Geometry: final body of the model. Coordinates: model frame, mm. A direction names the side the tool comes from. Coordinates: 2 decimals unless noted, no trailing zeros. Order: outer loops, then holes, each group sorted by start corner. A loop starts at its lowest first (then second) coordinate and runs counter-clockwise, first axis right, second up. Notation, with made-up numbers: (38, 22) - (69, 22) arc R30 ccw to (69, 48) - close; hole circle Ø11 at (-2, 83.5). An arc over 180 degrees is marked (long way). Use a Markdown table: item, result. Add a question column.
```python
from build123d import *

# Parameters (mm, degrees)
EXTRUDE1_DEPTH     = 1500
SKETCH2_R          = 13
CUT_EXTRUDE1_DEPTH = 10


with BuildPart() as part:
    # Sketch1 → Extrude1 (new body)
    with BuildSketch(Plane(origin=(0, 0, 0), x_dir=(0, 0, -1), z_dir=(1, 0, 0))):
        with BuildLine():
            Line((140, 10), (140, 100))
            Line((140, 100), (150, 100))
            Line((150, 100), (150, 10))
            ThreePointArc((150, 10), (147.071067812, 2.928932188), (140, 0))
            Line((140, 0), (10, 0))
            ThreePointArc((10, 0), (2.928932188, 2.928932188), (0, 10))
            Line((0, 10), (0, 100))
            Line((0, 100), (10, 100))
            Line((10, 100), (10, 10))
            Line((10, 10), (140, 10))
        make_face()
    extrude(amount=EXTRUDE1_DEPTH)

    # Sketch2 → Cut-Extrude1 (cut)
    with BuildSketch(Plane.XY):
        with Locations((225, 50)):
            Circle(SKETCH2_R)
        with Locations((1275, 50)):
            Circle(SKETCH2_R)
    extrude(amount=-CUT_EXTRUDE1_DEPTH, mode=Mode.SUBTRACT)


solid = part.part
```
1) Ray query, line 1 along Z through (x, y) = (1191, 67.5); line 2 along Y through (x, z) = (1268, -6); line 3 along Y through (x, z) = (225, -7). Return the intervals inside material, ascending.
2) Draft query along Z for faces 4 (the face through (740, 56, -150)), 5 (the face through (740, 10, -74)), 6 (the face through (212.013, 50.572, -4.93)). Return one class per face: pulls with the +Z half, pulls with the -Z half, needs draft (parallel to the pull), parting line crosses it, or undercut.
3) Section C-C (x = 780.5). Return loops of the section in (y, z), then the cut area to 3 significant figures.
4) Pin query (flat end, axial travel): pin 1 (8 mm diameter, centred on x = 1188, z = -49.5, fed in from +Y). Return the tip coordinate at first contact, or that it passes through.
5) Set-up query: faces 1 (the face through (1262.013, 50.572, -4.93)), 2 (the face through (740, 0, -76)), 3 (the face through (740, 56, -10)). Return all of +Z, -Z, +X, -X, +Y, -Y with unobstructed straight access to the full face (end or side cutting, diameter ignored); none if empty.
6) Section D-D (z = -69). Return loops of the section in (x, y), then the cut area to 3 significant figures.
7) Section A-A (x = 1275). Return loops of the section in (y, z), then the cut area to 3 significant figures.
8) Section B-B (y = 50). Return loops of the section in (x, z).
Values follow:
| question | item | result |
|---|---|---|
| 1 | line 1 | z = -150 to -140, -10 to 0 |
| 1 | line 2 | y = 0.83 to 39.05, 60.95 to 100 |
| 1 | line 3 | y = 0.46 to 37, 63 to 100 |
| 2 | face 4 | pulls with the -Z half |
| 2 | face 5 | undercut |
| 2 | face 6 | needs draft |
| 3 | outline | (0, -140) arc R10 ccw to (10, -150) - (100, -150) - (100, -140) - (10, -140) - (10, -10) - (100, -10) - (100, 0) - (10, 0) arc R10 ccw to (0, -10) - close |
| 3 | area | 3,260 mm² |
| 4 | pin 1 | stops at y = 10 |
| 5 | face 1 | +Z |
| 5 | face 2 | +Z, -Z, +X, -X, -Y |
| 5 | face 3 | +X, -X, +Y |
| 6 | outline | (0, 0) - (1500, 0) - (1500, 10) - (0, 10) - close |
| 6 | area | 15,000 mm² |
| 7 | outline | (0, -140) arc R10 ccw to (10, -150) - (100, -150) - (100, -140) - (10, -140) - (10, -10) - (37, -10) - (37, 0) - (10, 0) arc R10 ccw to (0, -10) - close; (63, -10) - (100, -10) - (100, 0) - (63, 0) - close |
| 7 | area | 3,000 mm² |
| 8 | outline | (0, -150) - (1500, -150) - (1500, -140) - (0, -140) - close; (0, -10) - (212, -10) - (212, 0) - (0, 0) - close; (238, -10) - (1262, -10) - (1262, 0) - (238, 0) - close; (1288, -10) - (1500, -10) - (1500, 0) - (1288, 0) - close |
